CAD build for the part. Positions are in the model's coordinates, mm. A direction names the side the tool comes from. Round coordinates to 2 decimals unless told otherwise and drop trailing zeros. Write each loop counter-clockwise with the first axis right and the second up, starting at its lowest first coordinate (ties: lowest second). Pieces come first, ordered by that corner, then holes. Notation, with made-up numbers: (58.25, -28) -> (99.25, -28) arc R14 cw to (99.25, -16) -> close; hole circle Ø3 at (-40, 11). An arc over 180 degrees is marked (long way). Answer in a Markdown table with one row per item. Add a question column.
```python
from build123d import *

# Parameters (mm, degrees)
SWEEP1_PROFILE_R   = 2.5
CUT_EXTRUDE1_DEPTH = 10


with BuildPart() as part:
    # Sweep1: sweep along a path in Sketch1
    with BuildLine(Plane(origin=(0, 0, 0), x_dir=(1, 0, 0), z_dir=(0, 1, 0))) as sweep1_path:
        Line((339.702814789, 0), (324.702814789, 0))
        Line((324.702814789, 0), (250.204561609, 0))
    # Sweep1 profile (on start of the path) → Sweep1 (sweep)
    with BuildSketch(Plane(origin=(339.702814789, 0, 0), x_dir=(0, 0, -1), z_dir=(-1, 0, 0))):
        Circle(SWEEP1_PROFILE_R)
    sweep(path=sweep1_path.line)

    # Sketch4 → Cut-Extrude1 (cut)
    with BuildSketch(Plane(origin=(250.204561609, 0, 0), x_dir=(0, 0, -1), z_dir=(-1, 0, 0))):
        with BuildLine():
            Line((-2.5, 0), (-0.194982329, 0))
            ThreePointArc((-0.194982329, 0), (-0.137873327, 0.137873327), (0, 0.194982329))
            Line((0, 0.194982329), (0, 2.5))
            ThreePointArc((0, 2.5), (1.767766953, 1.767766953), (2.5, 0))
            Line((2.5, 0), (0.194982329, 0))
            ThreePointArc((0.194982329, 0), (0.137873327, -0.137873327), (0, -0.194982329))
            Line((0, -0.194982329), (0, -2.5))
            ThreePointArc((0, -2.5), (-1.767766953, -1.767766953), (-2.5, 0))
        make_face()
    extrude(amount=-CUT_EXTRUDE1_DEPTH, mode=Mode.SUBTRACT)


solid = part.part
```
Item 1: Tool access for faces 1 (the flat face through (255, 0, 1)), 2 (the cylindrical face through (294.33, -1.69, 1.84)), 3 (the flat face through (255, -1, 0)), 4 (the flat face through (260.205, 0, 0)), 5 (the flat face through (250.205, 1, -1)): list every direction of +Z, -Z, +X, -X, +Y, -Y with a clear straight run to the whole face (end or side of a thin tool).
Item 2: Pin check, flat tips, straight feed: pin 1 (0.7 mm diameter, centred on x = 255, y = 1, fed in from +Z); pin 2 (1.2 mm diameter, centred on x = 254.5, z = -1.5, fed in from -Y); pin 3 (2 mm diameter, centred on x = 284, z = 1.5, fed in from -Y). Stop position of each tip, or through.
Item 3: Saw through at B-B on y = 1.35. Give the cut face in (x, z), then the cut area to 3 significant figures.
Item 4: Drill centre lines: probe 1 along Z at (x, y) = (288, 0.2); probe 2 along X at (y, z) = (0.1, 0.2); probe 3 along Y at (x, z) = (305, -2.25). Where is each one in solid material? Low to high.
Item 5: Saw through at A-A on z = -1.4. Give the cut face in (x, y), then the cut area to 3 significant figures.
Item 6: Saw through at C-C on x = 290. Give the cut face in (y, z), then the cut area to 3 significant figures.
Recorded:
| question | item | result |
|---|---|---|
| 1 | face 1 | +Z, -X, +Y |
| 1 | face 2 | +X, -X |
| 1 | face 3 | -Z, -X, -Y |
| 1 | face 4 | -X |
| 1 | face 5 | +Z, -Z, -X, +Y, -Y |
| 2 | pin 1 | z = 0 |
| 2 | pin 2 | y = 0 |
| 2 | pin 3 | y = -2.45 |
| 3 | outline | (250.2, -2.1) -> (339.7, -2.1) -> (339.7, 2.1) -> (260.2, 2.1) -> (260.2, 0) -> (250.2, 0) -> close |
| 3 | area | 356 mm2 |
| 4 | probe 1 | -2.49 to 2.49 |
| 4 | probe 2 | 260.2 to 339.7 |
| 4 | probe 3 | -1.09 to 1.09 |
| 5 | outline | (250.2, 0) -> (260.2, 0) -> (260.2, -2.07) -> (339.7, -2.07) -> (339.7, 2.07) -> (250.2, 2.07) -> close |
| 5 | area | 350 mm2 |
| 6 | outline | circle Ø5 at (0, 0) |
| 6 | area | 19.6 mm2 |
